Input: part model. Units: mm. Frame: model coordinates. A direction names the side the tool comes from. Round coordinates to 2 decimals unless told otherwise and drop trailing zeros. Loops run counter-clockwise (first coordinate to the right, second up) from the corner with the lowest first, then second, coordinate; pieces in that order, holes last. Notation, with made-up numbers: M 40,-26.5 L 98,-26.5 A24 ccw 98,12.5 Z; hole C -14,49 d4. An arc over 180 degrees is marked long. Put each result on its own line as item: value. Start each with the question number.
1) Pin query (flat end, axial travel): pin 1 (10 mm diameter, centred on y = 7, z = -9, fed in from +X); pin 2 (6 mm diameter, centred on x = 9.5, y = 13.5, fed in from -Z); pin 3 (1.5 mm diameter, centred on x = 16, z = 23.5, fed in from +Y). Return the tip coordinate at first contact, or that it passes through.
2) Draft query along X for faces 3 (the face through (-3, 8, 3)), 4 (the face through (10, 10, 0)), 5 (the face through (9.67, 1.52, 27.52)), 6 (the face through (0, 8, -12)). Return one class per face: +X half, -X half, draft (parallel to the pull), parting line (faces both ways), or undercut.
3) Section D-D on x = 1.5. Output: boundary loops of the cut face in (y, z), plus the area to 3 significant figures.
4) Line query: probe 1 along Z at (x, y) = (10, 2.45); probe 2 along Y at (x, z) = (-1.45, -10); probe 3 along X at (y, z) = (2.2, 30). Output: solid intervals per line, ascending.
5) Section B-B on y = 9.25. Output: boundary loops of the cut face in (x, z), plus the area to 3 significant figures.
6) Reachability of faces 1 (the face through (-2, 10, -20)), 2 (the face through (10, 11, 3)) from +Z, -Z, +X, -X, +Y, -Y: full face, straight path, thin tool, end or side. Return the list, or none.
7) Section C-C on z = -10. Output: boundary loops of the cut face in (x, y), plus the area to 3 significant figures.
8) Section A-A on x = 10. Output: boundary loops of the cut face in (y, z), plus the area to 3 significant figures.
from build123d import *

# Parameters (mm, degrees)
SKETCH1_W           = 3
SKETCH1_H           = 20
BOSS_EXTRUDE1_DEPTH = 20
SKETCH3_W           = 20
SKETCH3_H           = 40
BOSS_EXTRUDE2_DEPTH = 3
BOSS_EXTRUDE3_DEPTH = 3
SKETCH5_R           = 2.5
CUT_EXTRUDE1_DEPTH  = 3
SKETCH6_R           = 2.5
CUT_EXTRUDE2_DEPTH  = 3


with BuildPart() as part:
    # Sketch1 → Boss-Extrude1 (new body)
    with BuildSketch(Plane(origin=(0, 0, 0), x_dir=(1, 0, 0), z_dir=(0, 1, 0))):
        Polygon((20, 0), (0, 0), (-3, 0), (-3, -3), (20, -3), align=None)
        with Locations((-1.5, 10)):
            Rectangle(SKETCH1_W, SKETCH1_H)
    extrude(amount=BOSS_EXTRUDE1_DEPTH)

    # Sketch3 → Boss-Extrude2 (add)
    with BuildSketch(Plane.XZ):
        with Locations((10, 20)):
            Rectangle(SKETCH3_W, SKETCH3_H)
    extrude(amount=-BOSS_EXTRUDE2_DEPTH)

    # Sketch4 → Boss-Extrude3 (add)
    with BuildSketch(Plane.ZY.offset(3)):
        Polygon((3, 20), (3, 0), (40, 0), (40, 3), align=None)
    extrude(amount=-BOSS_EXTRUDE3_DEPTH)

    # Sketch5 → Cut-Extrude1 (cut)
    with BuildSketch(Plane(origin=(0, 0, 0), x_dir=(0, 0, -1), z_dir=(1, 0, 0))):
        with Locations((10, 10)):
            Circle(SKETCH5_R)
    extrude(amount=-CUT_EXTRUDE1_DEPTH, mode=Mode.SUBTRACT)

    # Sketch6 → Cut-Extrude2 (cut)
    with BuildSketch(Plane(origin=(0, 3, 0), x_dir=(1, 0, 0), z_dir=(0, 1, 0))):
        with Locations((10, -30)):
            Circle(SKETCH6_R)
    extrude(amount=-CUT_EXTRUDE2_DEPTH, mode=Mode.SUBTRACT)


solid = part.part
Geometry results:
1. pin 1: stops at x = 0
1. pin 2: stops at z = 0
1. pin 3: stops at y = 3
2. face 3: -X half
2. face 4: draft
2. face 5: undercut
2. face 6: +X half
3. outline: M 0,0 L 20,0 L 20,3 L 3,3 L 3,40 L 0,40 Z
3. area: 171 mm²
4. probe 1: z = 0 to 27.5, 32.5 to 40
4. probe 2: y = 0 to 7.5, 12.5 to 20
4. probe 3: x = -3 to 7.5, 12.5 to 20
5. outline: M -3,-20 L 0,-20 L 0,-12.38 L -3,-12.38 Z; M -3,-7.62 L 0,-7.62 L 0,0 L 20,0 L 20,3 L 0,3 L 0,26.4 L -3,26.4 Z
5. area: 185 mm²
6. face 1: -Z, +X, -X, +Y, -Y
6. face 2: +Z, +X, +Y
7. outline: M -3,0 L 0,0 L 0,7.5 L -3,7.5 Z; M -3,12.5 L 0,12.5 L 0,20 L -3,20 Z
7. area: 45.0 mm²
8. outline: M 0,0 L 20,0 L 20,3 L 3,3 L 3,27.5 L 0,27.5 Z; M 0,32.5 L 3,32.5 L 3,40 L 0,40 Z
8. area: 156 mm²
